from build123d import *

# Parameters (mm, degrees)
SKETCH_1_W               = 275
SKETCH_1_H               = 112
SKETCH_1_R               = 13
SKETCH_1_R_2             = 2.5
SKETCH_1_R_3             = 6.183267946
SKETCH_1_R_4             = 18
SKETCH_1_R_5             = 4
EXTRUDE_1_DEPTH          = 5
HOLE_WIZARD_M32_D        = 2.5
HOLE_WIZARD_M31_D        = 2.5
FILLET_1_R               = 2
HOLE_WIZARD_M35_D        = 2.5
PATTERN_CIRCULAR_1_COUNT = 4


with BuildPart() as part:
    # Эскиз1 → Бобышка-Вытянуть1 (new body)
    with BuildSketch(Plane.XY):
        with Locations((-40.858983849, 32)):
            Rectangle(SKETCH_1_W, SKETCH_1_H)
        Circle(SKETCH_1_R, mode=Mode.SUBTRACT)
        with Locations((-12.02081528, 12.02081528)):
            Circle(SKETCH_1_R_2, mode=Mode.SUBTRACT)
        with Locations((12.02081528, 12.02081528)):
            Circle(SKETCH_1_R_2, mode=Mode.SUBTRACT)
        with Locations((12.02081528, -12.02081528)):
            Circle(SKETCH_1_R_2, mode=Mode.SUBTRACT)
        with Locations((-12.02081528, -12.02081528)):
            Circle(SKETCH_1_R_2, mode=Mode.SUBTRACT)
        with Locations((-34.641016151, 20)):
            Circle(SKETCH_1_R_3, mode=Mode.SUBTRACT)
        with Locations((34.641016151, 20)):
            Circle(SKETCH_1_R_3, mode=Mode.SUBTRACT)
        with Locations((-116.358983849, 20)):
            Circle(SKETCH_1_R_4, mode=Mode.SUBTRACT)
        with Locations((-14.641016151, 78)):
            Circle(SKETCH_1_R_5, mode=Mode.SUBTRACT)
        with Locations((14.641016151, 78)):
            Circle(SKETCH_1_R_5, mode=Mode.SUBTRACT)
        with Locations((-96.358983849, 78)):
            Circle(SKETCH_1_R_5, mode=Mode.SUBTRACT)
    extrude(amount=EXTRUDE_1_DEPTH)

    # Отверстие обработанное метчиком M32 (through all)
    with Locations(Plane(origin=(0, 0, 0), x_dir=(-1, 0, 0), z_dir=(0, 0, -1))):
        with Locations((111.358983849, 57), (121.358983849, 57), (111.358983849, -17), (121.358983849, -17)):
            Hole(HOLE_WIZARD_M32_D / 2)

    # Отверстие обработанное метчиком M31 (through all)
    with Locations(Plane(origin=(-167.358983849, 71, 6), x_dir=(1, 0, 0), z_dir=(0, 0, 1))):
        with Locations((0, 0), (0, -10), (18, -10), (18, 0), (81.717967698, 0), (81.717967698, -10), (99.717967698, -10), (99.717967698, 0), (235, 0), (235, -10), (253, 0), (253, -10)):
            Hole(HOLE_WIZARD_M31_D / 2)

    # Скругление1
    fillet_1_edges = [part.edges().sort_by_distance(p)[0] for p in [
        (-178.358983849, 88, 2.5),
        (96.641016151, 88, 2.5),
        (96.641016151, -24, 2.5),
        (-178.358983849, -24, 2.5),
    ]]
    fillet(fillet_1_edges, radius=FILLET_1_R)

    # Отверстие обработанное метчиком M35 (through all)
    with Locations(Plane.XY.offset(5)):
        with Locations((-100.802634663, 35.556349186)):
            hole_wizard_m35 = Hole(HOLE_WIZARD_M35_D / 2)

    # Круговой массив1: Отверстие обработанное метчиком M35 ×4 about axis
    pattern_circular_1_axis = Axis((-116.358983849, 20, 0), (0, 0, 1))
    for i in range(1, PATTERN_CIRCULAR_1_COUNT):
        add(hole_wizard_m35.rotate(pattern_circular_1_axis, i * 360 / PATTERN_CIRCULAR_1_COUNT), mode=Mode.SUBTRACT)


solid = part.part
Work out the finished part from the listing and answer in its coordinate system (mm). Coordinates: 2 decimals unless noted, no trailing zeros. Loops run counter-clockwise (first coordinate to the right, second up) from the corner with the lowest first, then second, coordinate; pieces in that order, holes last. Notation, with made-up numbers: (-16.5, -3.75) -> (40.5, -3.75) arc R18 ccw to (40.5, 12.25) -> close; hole circle Ø7 at (9, 22). An arc over 180 degrees is marked (long way). Write each question's results on one line, items separated by ' | '. Start each with the question number.
1) The mould has two halves that part along Y. Classify faces 1 (the cylindrical face through (28.464, 20.272, 2.465)), 2 (the flat face through (96.641, 31, 2)), 3 (the flat face through (-43, 88, 2)): pulls with the +Y half, pulls with the -Y half, needs draft (parallel to the pull), parting line crosses it, or undercut.
2) Find section C-C on y = 20. Determine the outline of the cut face in (x, z).
3) Find section D-D on x = -128. Determine the outline of the cut face in (y, z), then the cut area to 3 significant figures.
4) Find section B-B on y = 78. Determine the outline of the cut face in (x, z), then the cut area to 4 significant figures.
5) A flat-ended cylindrical pin translates along its axis: P1, Ø21.5, axis at x = -116.36, y = 20, coming from the +Z side. Find the tip coordinate at first contact, or state that the pin passes through.
6) Find section A-A on x = 0. Determine the outline of the cut face in (y, z).
7) Consider line 1 along Y through (x, z) = (-67.5, 1.5); line 2 along Y through (x, z) = (10.5, 1.65); line 3 along X through (y, z) = (10, 3.95). Determine where each line is inside the solid, lowest interval first.
Response values:
1) face 1: undercut | face 2: needs draft | face 3: pulls with the +Y half
2) outline: (-178.36, 0) -> (-134.36, 0) -> (-134.36, 5) -> (-178.36, 5) -> close; (-98.36, 0) -> (-40.82, 0) -> (-40.82, 5) -> (-98.36, 5) -> close; (-28.46, 0) -> (28.46, 0) -> (28.46, 5) -> (-28.46, 5) -> close; (40.82, 0) -> (96.64, 0) -> (96.64, 5) -> (40.82, 5) -> close
3) outline: (-24, 0) -> (6.27, 0) -> (6.27, 5) -> (-24, 5) -> close; (33.73, 0) -> (88, 0) -> (88, 5) -> (33.73, 5) -> close | area: 423 mm^2
4) outline: (-178.36, 0) -> (-100.36, 0) -> (-100.36, 5) -> (-178.36, 5) -> close; (-92.36, 0) -> (-18.64, 0) -> (-18.64, 5) -> (-92.36, 5) -> close; (-10.64, 0) -> (10.64, 0) -> (10.64, 5) -> (-10.64, 5) -> close; (18.64, 0) -> (96.64, 0) -> (96.64, 5) -> (18.64, 5) -> close | area: 1,255 mm^2
5) P1: passes through
6) outline: (-24, 0) -> (-13, 0) -> (-13, 5) -> (-24, 5) -> close; (13, 0) -> (88, 0) -> (88, 5) -> (13, 5) -> close
7) line 1: y = -24 to 59.76, 62.24 to 69.76, 72.24 to 88 | line 2: y = -24 to -14.01, -10.04 to -7.66, 7.66 to 10.04, 14.01 to 88 | line 3: x = -178.36 to -131.33, -101.39 to -13.49, -10.55 to -8.31, 8.31 to 10.55, 13.49 to 96.64
